Geometry check sheet. Reference: the model listing, model coordinates, mm. Coordinates: 2 decimals unless noted, no trailing zeros. Loops run counter-clockwise (first coordinate to the right, second up) from the corner with the lowest first, then second, coordinate; pieces in that order, holes last. Notation, with made-up numbers: M 52,67.5 L 87,67.5 A14 cw 87,91.5 Z; hole C 11.5,-13.75 d10. An arc over 180 degrees is marked long. One line per question, with ' | ' between items. Start each with the question number.
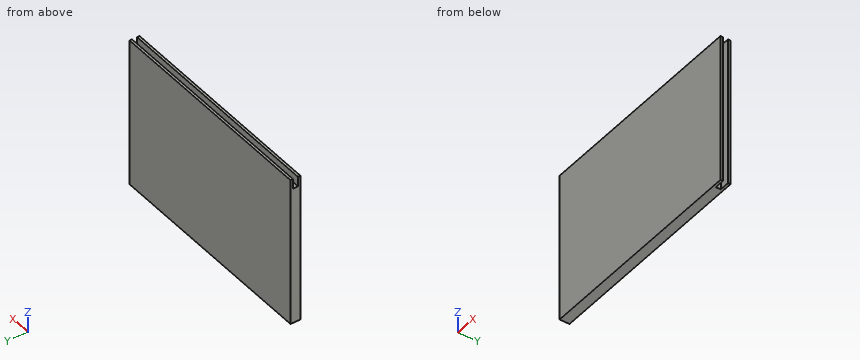
Autodesk Inventor part; units mm, degrees
ref_plane "YZ Plane" through (0, 0, 0) normal (1, 0, 0) x (0, 1, 0)
ref_plane "XZ Plane" through (0, 0, 0) normal (0, 1, 0) x (-1, 0, 0)
ref_plane "XY Plane" through (0, 0, 0) normal (0, 0, 1) x (1, 0, 0)
sketch "Sketch1" plane through (0, 0, 0) normal (0, 1, 0) x (-1, 0, 0)
  line L0 (-112.5, 75) -> (112.5, 75)
  line L1 (112.5, 75) -> (112.5, -75)
  line L2 (112.5, -75) -> (-112.5, -75)
  line L3 (-112.5, -75) -> (-112.5, 75)
  line L4 (-112.5, 75) -> (112.5, -75) construction
  line L5 (112.5, 75) -> (-112.5, -75) construction
  point P0 (0, 0)
  dimension "d0" = 225
  dimension "d1" = 150
extrude "Extrusion1" add sketch "Sketch1" along normal blind 10
sketch "Sketch4" plane through (112.5, 0, 75) normal (1, 0, 0) x (0, 0, -1)
  line L0 (0, 2.5) -> (150, 2.5)
  line L1 (150, 2.5) -> (150, 7.5)
  line L2 (150, 7.5) -> (0, 7.5)
  line L3 (0, 7.5) -> (0, 2.5)
  point P0 (75, 0)
  dimension "d12" = 150
  dimension "d13" = 5
extrude "Extrusion4" cut sketch "Sketch4" against normal blind 10
sketch "Sketch5" plane through (-112.5, 0, 75) normal (0, 0, 1) x (1, 0, 0)
  line L0 (0, 0) -> (0, 10)
  line L1 (0, 2.5) -> (225, 2.5)
  line L2 (225, 2.5) -> (225, 7.5)
  line L3 (225, 7.5) -> (0, 7.5)
  line L4 (0, 7.5) -> (0, 2.5)
  point P0 (112.5, 0)
  dimension "d16" = 225
  dimension "d17" = 5
extrude "Extrusion5" cut sketch "Sketch5" against normal blind 10
properties part number "TSU_Baseplate_Female"
1. Sectioned sample at A-A (z = 25.5). Record the cut outline in (x, y).
2. Depth check by flat-ended pin: pin 1 Ø4 at (y, z) = (4, -2.5) entering from +X; pin 2 Ø2.5 at (x, y) = (30.5, 4.5) entering from +Z. Enter the tip coordinate at first touch or a pass-through.
3. Sectioned sample at B-B (x = 30.5). Record the cut outline in (y, z).
4. Sectioned sample at C-C (y = 5). Record the cut outline in (x, z).
5. Thickness scan on line 1 (Z direction, x = 101.5, y = 5.75); line 2 (X direction, y = 5.5, z = 34.5). Record the ranges inside material, lowest first.
Result:
1) outline: M -112.5,0 L 112.5,0 L 112.5,2.5 L 102.5,2.5 L 102.5,7.5 L 112.5,7.5 L 112.5,10 L -112.5,10 Z
2) pin 1: stops at x = 112.5 | pin 2: stops at z = 65
3) outline: M 0,-75 L 10,-75 L 10,75 L 7.5,75 L 7.5,65 L 2.5,65 L 2.5,75 L 0,75 Z
4) outline: M -112.5,-75 L 102.5,-75 L 102.5,65 L -112.5,65 Z
5) line 1: z = -75 to 65 | line 2: x = -112.5 to 102.5
